```python
from build123d import *

# Parameters (mm, degrees)
SALIENTE_EXTRUIR1_DEPTH = 4
CROQUIS3_R              = 1.85
CORTAR_EXTRUIR1_DEPTH   = 5
REDONDEO1_R             = 5


with BuildPart() as part:
    # Croquis2 → Saliente-Extruir1 (new body)
    with BuildSketch(Plane(origin=(0, 0, -2.539999962), x_dir=(-1, 0, 0), z_dir=(0, 1, 0))):
        with BuildLine():
            Line((-157.5, 62.039999962), (-165, 62.039999962))
            Line((-165, 62.039999962), (-165, 67.539999962))
            Line((-165, 67.539999962), (0, 67.539999962))
            Line((0, 67.539999962), (0, 62.039999962))
            Line((0, 62.039999962), (-7.5, 62.039999962))
            ThreePointArc((-7.5, 62.039999962), (-9.5, 60.039999962), (-7.5, 58.039999962))
            Line((-7.5, 58.039999962), (0, 58.039999962))
            Line((0, 58.039999962), (0, 52.539999962))
            Line((0, 52.539999962), (-31.793786053, 39.370582579))
            ThreePointArc((-31.793786053, 39.370582579), (-34.687388848, 35.039999962), (-31.793786053, 30.709417344))
            Line((-31.793786053, 30.709417344), (0, 17.539999962))
            Line((0, 17.539999962), (0, 12.039999962))
            Line((0, 12.039999962), (-7.5, 12.039999962))
            ThreePointArc((-7.5, 12.039999962), (-9.5, 10.039999962), (-7.5, 8.039999962))
            Line((-7.5, 8.039999962), (0, 8.039999962))
            Line((0, 8.039999962), (0, 2.539999962))
            Line((0, 2.539999962), (-165, 2.539999962))
            Line((-165, 2.539999962), (-165, 8.039999962))
            Line((-165, 8.039999962), (-157.5, 8.039999962))
            ThreePointArc((-157.5, 8.039999962), (-155.5, 10.039999962), (-157.5, 12.039999962))
            Line((-157.5, 12.039999962), (-165, 12.039999962))
            Line((-165, 12.039999962), (-165, 17.539999962))
            Line((-165, 17.539999962), (-133.206213947, 30.709417344))
            ThreePointArc((-133.206213947, 30.709417344), (-130.312611152, 35.039999962), (-133.206213947, 39.370582579))
            Line((-133.206213947, 39.370582579), (-165, 52.539999962))
            Line((-165, 52.539999962), (-165, 58.039999962))
            Line((-165, 58.039999962), (-157.5, 58.039999962))
            ThreePointArc((-157.5, 58.039999962), (-155.5, 60.039999962), (-157.5, 62.039999962))
        make_face()
    extrude(amount=SALIENTE_EXTRUIR1_DEPTH)

    # Croquis3 → Cortar-Extruir1 (cut, through all)
    with BuildSketch(Plane(origin=(0, 4, 0), x_dir=(-1, 0, 0), z_dir=(0, 1, 0))):
        with Locations((-99.5, 57)):
            Circle(CROQUIS3_R)
        with Locations((-41.5, 57)):
            Circle(CROQUIS3_R)
        with Locations((-41.5, 8)):
            Circle(CROQUIS3_R)
        with Locations((-99.5, 8)):
            Circle(CROQUIS3_R)
        with Locations((-63.5, 42.5)):
            Circle(CROQUIS3_R)
        with Locations((-118.1, 17.1)):
            Circle(CROQUIS3_R)
    extrude(amount=-CORTAR_EXTRUIR1_DEPTH, mode=Mode.SUBTRACT)

    # Redondeo1
    redondeo1_edges = [part.edges().sort_by_distance(p)[0] for p in [
        (165, 2, 65),
        (0, 2, 65),
        (0, 2, 50),
        (0, 2, 15),
        (0, 2, 0),
        (165, 2, 0),
        (165, 2, 15),
        (165, 2, 50),
    ]]
    fillet(redondeo1_edges, radius=REDONDEO1_R)


solid = part.part
```
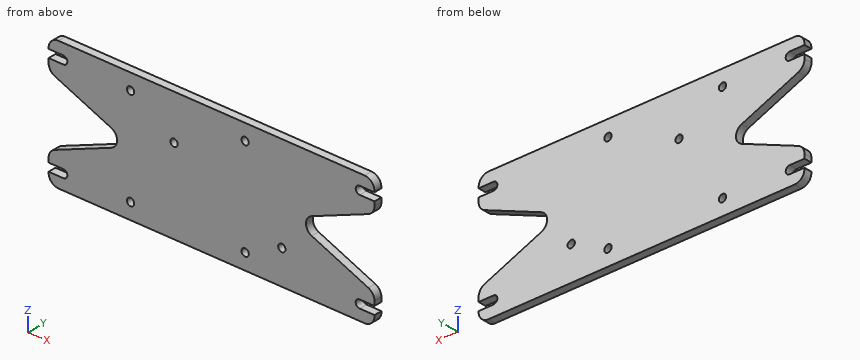
Verification items for the finished model (mm, model axes). Round coordinates to 2 decimals unless told otherwise and drop trailing zeros. Write each loop counter-clockwise with the first axis right and the second up, starting at its lowest first coordinate (ties: lowest second). Pieces come first, ordered by that corner, then holes.
1. Section check B-B on z = 42.5. Enter the section's corners in (x, y), plus the area to 3 significant figures.
2. Section check A-A on x = 99.5. Enter the section's corners in (y, z).
3. Gauge pin test, flat ends, axial feed: P1, Ø1.2, axis at x = 4, y = 2.5, coming from the +Z side; P2, Ø1.2, axis at x = 2, y = 2.5, coming from the +Z side; P3, Ø3, axis at x = 99.5, z = 8, coming from the +Y side; P4, Ø2, axis at x = 2.5, y = 2, coming from the -Z side. Record the tip position at first contact, or that the pin passes through.
4. Section check C-C on x = 136. Enter the section's corners in (y, z), plus the area to 3 significant figures.
5. Section check D-D on y = 1. State how many separate pieces and enclosed holes the cut face has, plus the area to 3 significant figures.
6. Scan lines: L1, parallel to Z at x = 41.5, y = 2.95; L2, parallel to Z at x = 118.1, y = 1.7; L3, parallel to Z at x = 34, y = 1. Record each from-to range of solid material in increasing order.
Answer:
1. outline: (18.11, 0) - (61.65, 0) - (61.65, 4) - (18.11, 4) - close; (65.35, 0) - (146.89, 0) - (146.89, 4) - (65.35, 4) - close
1. area: 500 mm2
2. outline: (0, 0) - (4, 0) - (4, 6.15) - (0, 6.15) - close; (0, 9.85) - (4, 9.85) - (4, 55.15) - (0, 55.15) - close; (0, 58.85) - (4, 58.85) - (4, 65) - (0, 65) - close
3. P1: stops at z = 64.98
3. P2: stops at z = 64.39
3. P3: passes through
3. P4: stops at z = 0.23
4. outline: (0, 0) - (4, 0) - (4, 27.01) - (0, 27.01) - close; (0, 37.99) - (4, 37.99) - (4, 65) - (0, 65) - close
4. area: 216 mm2
5. separate pieces: 1
5. enclosed holes: 6
5. area: 9,060 mm2
6. L1: z = 0 to 6.15, 9.85 to 55.15, 58.85 to 65
6. L2: z = 0 to 15.25, 18.95 to 65
6. L3: z = 0 to 30.06, 34.94 to 65
